Design review of the part built by this model. Coordinates are the model's own, in mm. A direction names the side the tool comes from. Give positions to 0.01 mm unless a question says otherwise; leave off trailing zeros. Order: outer loops, then holes, each group sorted by start corner. A loop starts at its lowest first (then second) coordinate and runs counter-clockwise, first axis right, second up. Notation, with made-up numbers: (21, -3) -> (68, -3) arc R31 ccw to (68, 27) -> close; hole circle Ø2 at (2.25, -19). An arc over 180 degrees is marked (long way). Return JSON: item names as keys, results as strings.
```python
from build123d import *

# Parameters (mm, degrees)
SKETCH1_R           = 41
BOSS_EXTRUDE1_DEPTH = 10
SKETCH2_R           = 10.1
CUT_EXTRUDE1_DEPTH  = 0.5
SKETCH3_R           = 1.7
SKETCH3_R_2         = 2
CUT_EXTRUDE2_DEPTH  = 59.755850772
SKETCH4_R           = 3.25
CUT_EXTRUDE3_DEPTH  = 3
SKETCH5_R           = 2.1
CUT_EXTRUDE4_DEPTH  = 5.5


with BuildPart() as part:
    # Sketch1 → Boss-Extrude1 (new body)
    with BuildSketch(Plane(origin=(0, 0, 0), x_dir=(1, 0, 0), z_dir=(0, 1, 0))):
        with Locations(Location((0, 0, 0), (0, 0, 270))):
            Circle(SKETCH1_R)
    extrude(amount=BOSS_EXTRUDE1_DEPTH)

    # Sketch2 → Cut-Extrude1 (cut)
    with BuildSketch(Plane.XZ):
        with Locations(Location((0, 0, 0), (0, 0, 270))):
            Circle(SKETCH2_R)
    extrude(amount=-CUT_EXTRUDE1_DEPTH, mode=Mode.SUBTRACT)

    # Sketch3 → Cut-Extrude2 (cut, through all)
    with BuildSketch(Plane.XZ.offset(-0.5)):
        with Locations(Location((0, 7, 0), (0, 0, 270))):
            Circle(SKETCH3_R)
        with Locations(Location((7, 0, 0), (0, 0, 270))):
            Circle(SKETCH3_R)
        with Locations(Location((0, -7, 0), (0, 0, 270))):
            Circle(SKETCH3_R)
        with Locations(Location((-7, 0, 0), (0, 0, 270))):
            Circle(SKETCH3_R)
        with Locations(Location((0, 0, 0), (0, 0, 270))):
            Circle(SKETCH3_R_2)
    extrude(amount=-CUT_EXTRUDE2_DEPTH, mode=Mode.SUBTRACT)

    # Sketch4 → Cut-Extrude3 (cut)
    with BuildSketch(Plane(origin=(0, 10, 0), x_dir=(1, 0, 0), z_dir=(0, 1, 0))):
        with Locations(Location((0, 7, 0), (0, 0, 270))):
            Circle(SKETCH4_R)
        with Locations(Location((7, 0, 0), (0, 0, 270))):
            Circle(SKETCH4_R)
        with Locations(Location((0, -7, 0), (0, 0, 270))):
            Circle(SKETCH4_R)
        with Locations(Location((-7, 0, 0), (0, 0, 270))):
            Circle(SKETCH4_R)
    extrude(amount=-CUT_EXTRUDE3_DEPTH, mode=Mode.SUBTRACT)

    # Sketch5 → Cut-Extrude4 (cut)
    with BuildSketch(Plane(origin=(0, 10, 0), x_dir=(1, 0, 0), z_dir=(0, 1, 0))):
        with Locations(Location((-30, 15, 0), (0, 0, 270))):
            Circle(SKETCH5_R)
        with Locations(Location((-30, -15, 0), (0, 0, 270))):
            Circle(SKETCH5_R)
        with Locations(Location((30, 15, 0), (0, 0, 270))):
            Circle(SKETCH5_R)
        with Locations(Location((30, -15, 0), (0, 0, 270))):
            Circle(SKETCH5_R)
    extrude(amount=-CUT_EXTRUDE4_DEPTH, mode=Mode.SUBTRACT)


solid = part.part
```
Item 1: Mouldability with a two-part tool opening along X and no side actions: class faces 4 (the face through (30, 4.5, 15)), 5 (the face through (-40, 5, -9)), 6 (the face through (-9, 0, 9)) as released by +X, released by -X, zero draft, split by the parting line, or undercut.
Result set:
{"face 4": "undercut", "face 5": "split by the parting line", "face 6": "zero draft"}
Item 2: For pin 1 (6 mm diameter, centred on x = 1.5, z = 3, fed in from -Y); pin 2 (1.5 mm diameter, centred on x = -30.5, y = 7, fed in from +Z); pin 3 (5 mm diameter, centred on x = 7, z = 0.5, fed in from +Y), all flat-tipped, find the tip position at first contact; note any pin that passes through.
Result set:
{"pin 1": "stops at y = 0.5", "pin 2": "stops at z = 28.21", "pin 3": "stops at y = 7"}
Item 3: Add section B-B (x = 0). Give the boundary of the cut face in (y, z), plus the area to 3 significant figures.
Result set:
{"outline": "(0, -41) -> (10, -41) -> (10, -10.25) -> (7, -10.25) -> (7, -8.7) -> (0.5, -8.7) -> (0.5, -10.1) -> (0, -10.1) -> close; (0, 10.1) -> (0.5, 10.1) -> (0.5, 8.7) -> (7, 8.7) -> (7, 10.25) -> (10, 10.25) -> (10, 41) -> (0, 41) -> close; (0.5, -5.3) -> (7, -5.3) -> (7, -3.75) -> (10, -3.75) -> (10, -2) -> (0.5, -2) -> close; (0.5, 2) -> (10, 2) -> (10, 3.75) -> (7, 3.75) -> (7, 5.3) -> (0.5, 5.3) -> close", "area": "689 mm^2"}
Item 4: Add section A-A (y = 8.5). Give the number of separate pieces and of enclosed holes in the cut face, plus the area to 3 significant figures.
Result set:
{"separate pieces": "1", "enclosed holes": "9", "area": "5,080 mm^2"}
Item 5: Add section C-C (z = -15). Give the boundary of the cut face in (x, y), plus the area to 3 significant figures.
Result set:
{"outline": "(-38.16, 0) -> (38.16, 0) -> (38.16, 10) -> (32.1, 10) -> (32.1, 4.5) -> (27.9, 4.5) -> (27.9, 10) -> (-27.9, 10) -> (-27.9, 4.5) -> (-32.1, 4.5) -> (-32.1, 10) -> (-38.16, 10) -> close", "area": "717 mm^2"}
Item 6: Add section D-D (x = -30). Give the boundary of the cut face in (y, z), plus the area to 3 significant figures.
Result set:
{"outline": "(0, -27.95) -> (10, -27.95) -> (10, -17.1) -> (4.5, -17.1) -> (4.5, -12.9) -> (10, -12.9) -> (10, 12.9) -> (4.5, 12.9) -> (4.5, 17.1) -> (10, 17.1) -> (10, 27.95) -> (0, 27.95) -> close", "area": "513 mm^2"}
Item 7: Machinability: for faces 1 (the face through (5.6, 7, 1.4)), 2 (the face through (5.34, 3.7, 0.37)), 3 (the face through (2.4, 0.5, 0.1)), which of the approach directions +Z, -Z, +X, -X, +Y, -Y give a long, thin tool a straight path to every point of the face, cutting with its end or side? Answer none if there is none.
Result set:
{"face 1": "+Y", "face 2": "+Y, -Y", "face 3": "-Y"}
Item 8: Wall thickness on L1, parallel to X at y = 5.5, z = 0; L2, parallel to X at y = 5.5, z = 15; L3, parallel to X at y = 4.25, z = -14: over which ranges is each line inside the solid? List them lowest first. Write a range as [from, to].
Result set:
{"L1": "x = [-41, -8.7], [-5.3, -2], [2, 5.3], [8.7, 41]", "L2": "x = [-38.16, -32.1], [-27.9, 27.9], [32.1, 38.16]", "L3": "x = [-38.54, 38.54]"}
